For this review, take the finished solid that the model builds, in its own axes (mm). A direction names the side the tool comes from. Give positions to 0.01 mm unless a question says otherwise; leave off trailing zeros. Write each loop counter-clockwise with the first axis right and the second up, starting at its lowest first coordinate (ties: lowest second). Pieces come first, ordered by that corner, then holes. Notation, with made-up numbers: (-30.75, 7.5) -> (21.25, 7.5) arc R22 cw to (21.25, 16.5) -> close; hole circle Ø5 at (81, 36.25). An arc over 180 degrees is marked (long way). Return JSON: item names as keys, results as strings.
from build123d import *

# Parameters (mm, degrees)
SKETCH1_R           = 6.35
BOSS_EXTRUDE1_DEPTH = 65.6
SKETCH2_R           = 3.175
INNER_CHAMBER_DEPTH = 60
SKETCH4_R           = 6.35
HEAD_DEPTH          = 8
HEAD_TAPER          = 5
FILLET1_R           = 2
SKETCH5_R           = 0.5
CUT_EXTRUDE2_DEPTH  = 8


with BuildPart() as part:
    # Sketch1 → Boss-Extrude1 (new body)
    with BuildSketch(Plane(origin=(0, 0, 0), x_dir=(1, 0, 0), z_dir=(0, 1, 0))):
        with Locations(Location((0, 0, 0), (0, 0, 270))):
            Circle(SKETCH1_R)
    extrude(amount=BOSS_EXTRUDE1_DEPTH)

    # Sketch2 → Inner Chamber (cut)
    with BuildSketch(Plane(origin=(0, 65.6, 0), x_dir=(1, 0, 0), z_dir=(0, 1, 0))):
        with Locations(Location((0, 0, 0), (0, 0, 270))):
            Circle(SKETCH2_R)
    extrude(amount=-INNER_CHAMBER_DEPTH, mode=Mode.SUBTRACT)

    # Sketch4 → Head (add)
    with BuildSketch(Plane.XZ):
        with Locations(Location((0, 0, 0), (0, 0, 270))):
            Circle(SKETCH4_R)
    extrude(amount=HEAD_DEPTH, taper=HEAD_TAPER)

    # Fillet1
    fillet1_edges = [part.edges().sort_by_distance(p)[0] for p in [
        (0, -8, 5.650090692),
    ]]
    fillet(fillet1_edges, radius=FILLET1_R)

    # Sketch5 → Cut-Extrude2 (cut)
    with BuildSketch(Plane.XY):
        with Locations((0, -5)):
            Circle(SKETCH5_R)
    extrude(amount=-CUT_EXTRUDE2_DEPTH, mode=Mode.SUBTRACT)


solid = part.part
1. For pin 1 (1.5 mm diameter, centred on y = 39, z = 4, fed in from -X); pin 2 (2 mm diameter, centred on y = 3.5, z = -2, fed in from +X); pin 3 (1.9 mm diameter, centred on x = -0.5, z = -0.5, fed in from +Y), all flat-tipped, find the tip position at first contact; note any pin that passes through.
Results found:
{"pin 1": "stops at x = -5.46", "pin 2": "stops at x = 6.27", "pin 3": "stops at y = 5.6"}
2. To check wall thickness, follow probe 1 along X at (y, z) = (39, -0.25); probe 2 along Y at (x, z) = (0, -1.3); probe 3 along Y at (x, z) = (0.5, 2.75). State the ranges of each line that lie inside material, in increasing order.
Results found:
{"probe 1": "x = -6.35 to -3.17, 3.17 to 6.35", "probe 2": "y = -8 to -5.5, -4.5 to 5.6", "probe 3": "y = -8 to 5.6"}
3. Add section A-A, the plane y = 30.5. State the section outline as (x, z) points (3 decimals).
Results found:
{"outline": "circle Ø12.7 at (0, 0); hole circle Ø6.35 at (0, 0)"}
4. For faces 4 (the conical face through (-5.873, -3.816, 1.304)), 5 (the cylindrical face through (-1.93, 36.02, -2.52)), list the 3-axis set-ups (+Z, -Z, +X, -X, +Y, -Y) from which the entire face can be reached by the end or side of a thin tool; tool diameter is ignored.
Results found:
{"face 4": "-Y", "face 5": "+Y"}
5. The part is to be moulded in two halves that separate along Z. For faces 1 (the flat face through (0, -8, 0)), 2 (the flat face through (0, 5.6, 0)), 3 (the cylindrical face through (-3.86, 32.34, -5.04)), say which applies: +Z half, -Z half, draft (parallel to the pull), parting line (faces both ways), or undercut.
Results found:
{"face 1": "draft", "face 2": "undercut", "face 3": "parting line"}
